The drawing under review shows one solid part. Ordinate dimensions are in mm from its lowest x, y, z. A direction names the side the tool comes from. Give positions to 0.01 mm unless a question says otherwise; leave off trailing zeros. Write each loop counter-clockwise with the first axis right and the second up, starting at its lowest first coordinate (ties: lowest second). Pieces come first, ordered by that corner, then holes. Notation, with made-up numbers: (-1, -4) -> (12, -4) arc R17 cw to (12, 18) -> close; hole circle Ø6 at (69.25, 40.25). An arc over 180 degrees is marked (long way). Put each result on its own line as item: value. Start each with the question number.
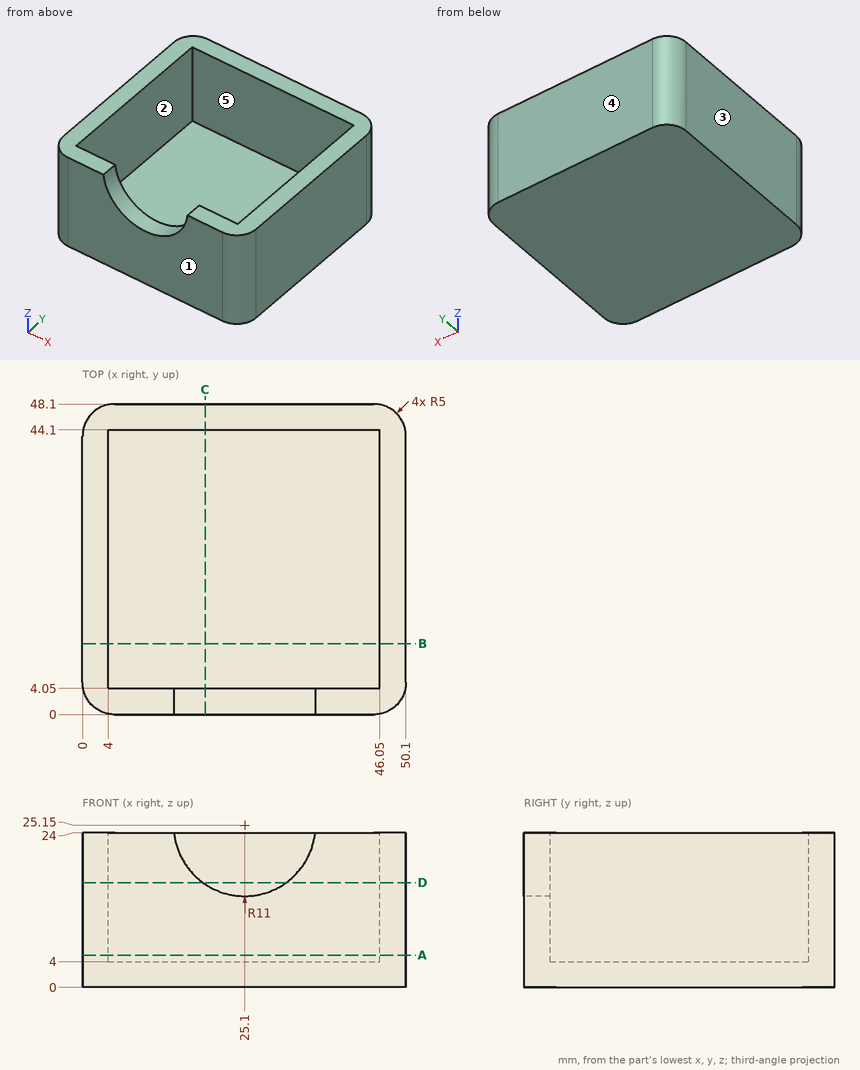
Q1. Take a section at D-D on z = 16.25. Give the boundary of the cut face in (x, y).
Q2. Take a section at C-C on x = 19. Give the boundary of the cut face in (y, z).
Q3. Machinability: for the marked faces 4 and 5, which of the approach directions +Z, -Z, +X, -X, +Y, -Y give a long, thin tool a straight path to every point of the face, cutting with its end or side? Answer none if there is none.
Q4. For pin 1 (12 mm diameter, centred on x = 22.5, y = 27.5, fed in from +Z), flat-tipped, find the tip position at first contact; note if it passes through.
Q5. Take a section at B-B on y = 11. Give the boundary of the cut face in (x, z), then the cut area to 3 significant figures.
Q6. Take a section at A-A on z = 5. Give the boundary of the cut face in (x, y).
Q7. Mouldability with a two-part tool opening along Y and no side actions: class the marked faces 1, 2 and 3 as +Y half, -Y half, draft (parallel to the pull), parting line (faces both ways), or undercut.
Q8. To check wall thickness, follow probe 1 along Y at (x, z) = (11, 6.75); probe 2 along X at (y, z) = (19, 19.25); probe 3 along Z at (x, y) = (15.5, 20). State the ranges of each line that lie inside material, in increasing order. Write a range as from..to.
Result:
1. outline: (0, 5) arc R5 ccw to (5, 0) -> (18.64, 0) -> (18.64, 4.05) -> (4, 4.05) -> (4, 44.1) -> (46.05, 44.1) -> (46.05, 4.05) -> (31.56, 4.05) -> (31.56, 0) -> (45.1, 0) arc R5 ccw to (50.1, 5) -> (50.1, 43.1) arc R5 ccw to (45.1, 48.1) -> (5, 48.1) arc R5 ccw to (0, 43.1) -> close
2. outline: (0, 0) -> (48.1, 0) -> (48.1, 24) -> (44.1, 24) -> (44.1, 4) -> (4.05, 4) -> (4.05, 16) -> (0, 16) -> close
3. face 4: +Z, -Z, +X, -X, +Y
3. face 5: +Z
4. pin 1: stops at z = 4
5. outline: (0, 0) -> (50.1, 0) -> (50.1, 24) -> (46.05, 24) -> (46.05, 4) -> (4, 4) -> (4, 24) -> (0, 24) -> close
5. area: 361 mm^2
6. outline: (0, 5) arc R5 ccw to (5, 0) -> (45.1, 0) arc R5 ccw to (50.1, 5) -> (50.1, 43.1) arc R5 ccw to (45.1, 48.1) -> (5, 48.1) arc R5 ccw to (0, 43.1) -> close; hole (4, 4.05) -> (46.05, 4.05) -> (46.05, 44.1) -> (4, 44.1) -> close
7. face 1: -Y half
7. face 2: undercut
7. face 3: draft
8. probe 1: y = 0..4.05, 44.1..48.1
8. probe 2: x = 0..4, 46.05..50.1
8. probe 3: z = 0..4
